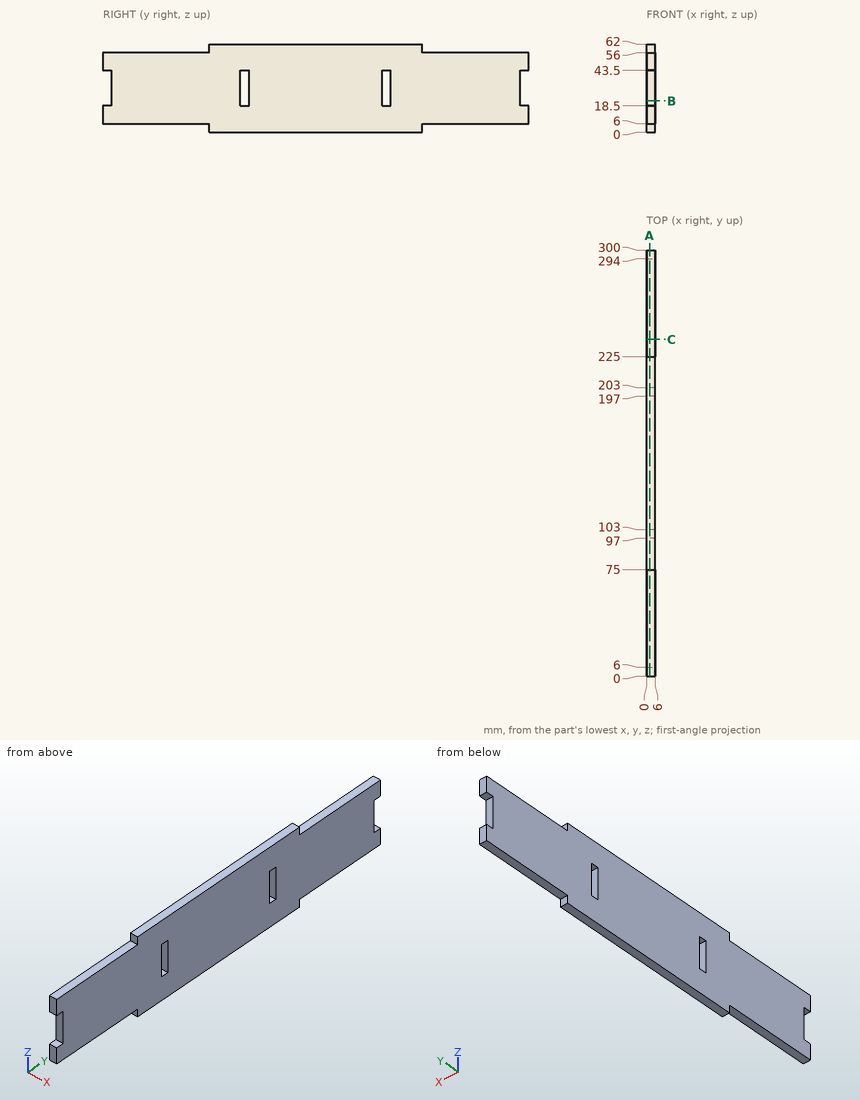
Verification items for this drawing (mm, ordinates from the low corner). Give positions to 0.01 mm unless a question says otherwise; leave off trailing zeros. Write each loop counter-clockwise with the first axis right and the second up, starting at its lowest first coordinate (ties: lowest second). Pieces come first, ordered by that corner, then holes.
1) Cross-section at C-C (y = 237). Record the boundary of the cut face in (x, z), plus the area to 3 significant figures.
Values follow:
outline: (0, 6) - (6, 6) - (6, 56) - (0, 56) - close
area: 300 mm2
2) Cross-section at A-A (x = 2). Record the boundary of the cut face in (y, z).
Values follow:
outline: (0, 6) - (75, 6) - (75, 0) - (225, 0) - (225, 6) - (300, 6) - (300, 18.5) - (294, 18.5) - (294, 43.5) - (300, 43.5) - (300, 56) - (225, 56) - (225, 62) - (75, 62) - (75, 56) - (0, 56) - (0, 43.5) - (6, 43.5) - (6, 18.5) - (0, 18.5) - close; hole (97, 18.5) - (103, 18.5) - (103, 43.5) - (97, 43.5) - close; hole (197, 18.5) - (203, 18.5) - (203, 43.5) - (197, 43.5) - close
3) Cross-section at B-B (z = 22). Record the boundary of the cut face in (x, y).
Values follow:
outline: (0, 6) - (6, 6) - (6, 97) - (0, 97) - close; (0, 103) - (6, 103) - (6, 197) - (0, 197) - close; (0, 203) - (6, 203) - (6, 294) - (0, 294) - close
4) Thickness scan on line 1 (Y direction, x = 1.8, z = 39); line 2 (Z direction, x = 5.35, y = 47). Record the ranges inside material, lowest first.
Values follow:
line 1: y = 6 to 97, 103 to 197, 203 to 294
line 2: z = 6 to 56
5) Go/stop test with flat-tipped pins: pin 1 Ø1.8 at (x, y) = (4, 45) entering from +Z; pin 2 Ø1.8 at (x, z) = (2.5, 36) entering from +Y. Record where each tip stops, or that it passes through.
Values follow:
pin 1: stops at z = 56
pin 2: stops at y = 294
